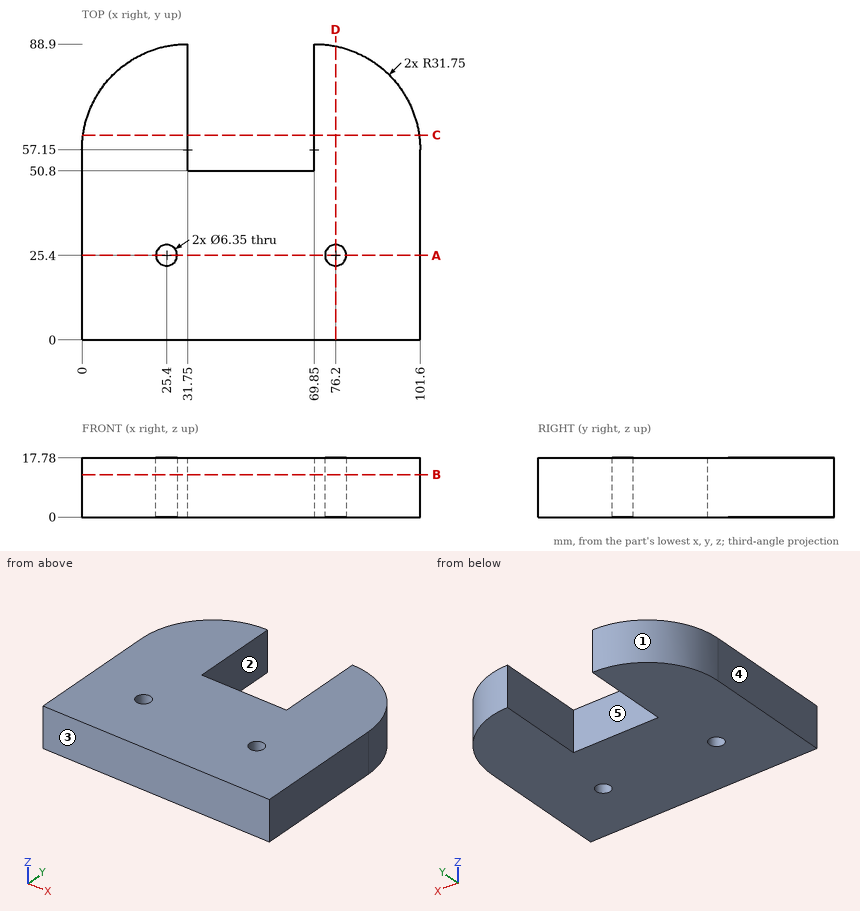
Part print with two shaded views. Sizes in mm from the minimum x, y, z corner. A direction names the side the tool comes from. Give positions to 0.01 mm unless a question says otherwise; leave off trailing zeros. Order: outer loops, then holes, each group sorted by start corner. A loop starts at its lowest first (then second) coordinate and runs counter-clockwise, first axis right, second up. Notation, with made-up numbers: M 19,55 L 39,55 A6 cw 39,61 Z; hole C 23,80 d5. An arc over 180 degrees is marked long. Put each result on its own line as item: value.
Item 1: Cut at A-A on y = 25.4. Write the cut outline in (x, z) (3 decimals).
Results are:
outline: M 0,0 L 22.225,0 L 22.225,17.78 L 0,17.78 Z; M 28.575,0 L 73.025,0 L 73.025,17.78 L 28.575,17.78 Z; M 79.375,0 L 101.6,0 L 101.6,17.78 L 79.375,17.78 Z
Item 2: Cut at D-D on x = 76.2. Write the cut outline in (y, z) (3 decimals), then the cut area to 3 significant figures.
Results are:
outline: M 0,0 L 22.225,0 L 22.225,17.78 L 0,17.78 Z; M 28.575,0 L 88.259,0 L 88.259,17.78 L 28.575,17.78 Z
area: 1,460 mm2
Item 3: Cut at B-B on z = 12.75. Write the cut outline in (x, y) (3 decimals).
Results are:
outline: M 0,0 L 101.6,0 L 101.6,57.15 A31.75 ccw 69.85,88.9 L 69.85,50.8 L 31.75,50.8 L 31.75,88.9 A31.75 ccw 0,57.15 Z; hole C 25.4,25.4 d6.35; hole C 76.2,25.4 d6.35
Item 4: Which spindle directions (+Z, -Z, +X, -X, +Y, -Y) get a long thin tool onto all of the face, cutting with end or side? Do the marked faces 1 and 2. Say none if no direction does.
Results are:
face 1: +Z, -Z, -X, +Y
face 2: +Z, -Z, +Y
Item 5: Drop flat-ended pins along their axis: pin 1 Ø1.5 at (y, z) = (73.5, 2.5) entering from +X; pin 2 Ø9 at (x, z) = (47.5, 12) entering from +Y. Give the stop position or say it passes through.
Results are:
pin 1: x = 97.5
pin 2: y = 50.8
Item 6: Pull direction X, two halves, no side cores. Call the marked faces 3, 4 and 5: +X half, -X half, draft (parallel to the pull), parting line (faces both ways), or undercut.
Results are:
face 3: draft
face 4: -X half
face 5: undercut
Item 7: Wall check: probe 1 along X at (y, z) = (84.5, 16.75); probe 2 along X at (y, z) = (63, 2.5); probe 3 along Y at (x, z) = (25.4, 4.5) (3 decimals). Give the ranges that are in metal, low to high.
Results are:
probe 1: 15.62 to 31.75, 69.85 to 85.98
probe 2: 0.54 to 31.75, 69.85 to 101.06
probe 3: 0 to 22.225, 28.575 to 88.259
Item 8: Cut at C-C on y = 61.5. Write the cut outline in (x, z), then the cut area to 3 significant figures.
Results are:
outline: M 0.3,0 L 31.75,0 L 31.75,17.78 L 0.3,17.78 Z; M 69.85,0 L 101.3,0 L 101.3,17.78 L 69.85,17.78 Z
area: 1,120 mm2
